```python
from build123d import *

# Parameters (mm, degrees)
BOSS_EXTRUDE1_DEPTH = 20
FILLET1_R           = 0.2
SKETCH2_R           = 2.7
CUT_EXTRUDE1_DEPTH  = 3.2
SKETCH3_R           = 2.7
CUT_EXTRUDE2_DEPTH  = 3.2


with BuildPart() as part:
    # Sketch1 → Boss-Extrude1 (new body)
    with BuildSketch(Plane.XY):
        with BuildLine():
            Line((5.679190751, 0), (19, 0))
            ThreePointArc((19, 0), (19.707106781, 0.292893219), (20, 1))
            Line((20, 1), (20, 2.2))
            ThreePointArc((20, 2.2), (19.707106781, 2.907106781), (19, 3.2))
            Line((19, 3.2), (5.2, 3.2))
            ThreePointArc((5.2, 3.2), (3.785786438, 3.785786438), (3.2, 5.2))
            Line((3.2, 5.2), (3.2, 19))
            ThreePointArc((3.2, 19), (2.907106781, 19.707106781), (2.2, 20))
            Line((2.2, 20), (1, 20))
            ThreePointArc((1, 20), (0.292893219, 19.707106781), (0, 19))
            Line((0, 19), (0, 2))
            ThreePointArc((0, 2), (0.585786438, 0.585786438), (2, 0))
            Line((2, 0), (5.679190751, 0))
        make_face()
    extrude(amount=BOSS_EXTRUDE1_DEPTH)

    # Fillet1
    fillet1_edges = [part.edges().sort_by_distance(p)[0] for p in [
        (2.907106781, 19.707106781, 20),
        (12.1, 3.2, 0),
        (19.707106781, 2.907106781, 0),
        (20, 1.6, 0),
        (19.707106781, 0.292893219, 0),
        (10.5, 0, 0),
        (0.585786438, 0.585786438, 0),
        (0, 10.5, 0),
        (0.292893219, 19.707106781, 0),
        (1.6, 20, 0),
        (1.6, 20, 20),
        (2.907106781, 19.707106781, 0),
        (3.2, 12.1, 0),
        (3.785786438, 3.785786438, 0),
        (0.292893219, 19.707106781, 20),
        (0, 10.5, 20),
        (0.585786438, 0.585786438, 20),
        (10.5, 0, 20),
        (19.707106781, 0.292893219, 20),
        (20, 1.6, 20),
        (19.707106781, 2.907106781, 20),
        (3.785786438, 3.785786438, 20),
        (12.1, 3.2, 20),
        (3.2, 12.1, 20),
    ]]
    fillet(fillet1_edges, radius=FILLET1_R)

    # Sketch2 → Cut-Extrude1 (cut)
    with BuildSketch(Plane.ZY):
        with Locations((10, 10)):
            Circle(SKETCH2_R)
    extrude(amount=-CUT_EXTRUDE1_DEPTH, mode=Mode.SUBTRACT)

    # Sketch3 → Cut-Extrude2 (cut)
    with BuildSketch(Plane.XZ):
        with Locations(Location((10, 10, 0), (0, 0, 270))):
            Circle(SKETCH3_R)
    extrude(amount=-CUT_EXTRUDE2_DEPTH, mode=Mode.SUBTRACT)


solid = part.part
```
Can you work these out from the model? Positions are in its coordinate system, mm. A direction names the side the tool comes from. Coordinates: 2 decimals unless noted, no trailing zeros. Loops run counter-clockwise (first coordinate to the right, second up) from the corner with the lowest first, then second, coordinate; pieces in that order, holes last. Notation, with made-up numbers: (20, 73.25) -> (26, 73.25) arc R13 cw to (26, 79.25) -> close; hole circle Ø9 at (-35, 74). An arc over 180 degrees is marked (long way). Put each result on its own line as item: value. Start each with the question number.
Q1. For faces 4 (the face through (14, 3.2, 10)), 5 (the face through (19.699, 0.285, 9.863)), which set-ups out of +Z, -Z, +X, -X, +Y, -Y let a thin tool reach every point of the face, with its end or its side?
Q2. I'm going to push flat-ended pins straight in: P1, Ø4.5, axis at y = 10, z = 10, coming from the -X side; P2, Ø2, axis at x = 11, z = 16.5, coming from the +Y side; P3, Ø5, axis at y = 17, z = 12.5, coming from the -X side; P4, Ø11, axis at y = 14.5, z = 12, coming from the +X side. Where does each tip first touch, or does it pass through?
Q3. I want a section at C-C (z = 10). Write out the boundary of the cut face in (x, y), plus the area to 3 significant figures.
Q4. I want a section at A-A (y = 10). Write out the boundary of the cut face in (x, z), plus the area to 3 significant figures.
Q5. I want a section at D-D (x = 7). Write out the boundary of the cut face in (y, z).
Q6. If I drill on line 1 (Y direction, x = 2.2, z = 10); line 2 (X direction, y = 11, z = 16), over which ranges is the centre line in solid material (lowest first)? Write a range as [from, to].
Q7. Thinking about a two-plate mould opening in X: for faces 1 (the face through (12.277, 1.578, 8.548)), 2 (the face through (2, 20, 10)), 3 (the face through (0.57, 0.6, 9.86)), which applies, pulls with the +X half, pulls with the -X half, needs draft (parallel to the pull), parting line crosses it, or undercut?
Taken from the geometry:
1. face 4: +Z, -Z, +X, +Y
1. face 5: +Z, -Z, +X, -Y
2. P1: passes through
2. P2: stops at y = 3.2
2. P3: stops at x = 0
2. P4: stops at x = 3.2
3. outline: (0, 2) arc R2 ccw to (2, 0) -> (7.3, 0) -> (7.3, 3.2) -> (5.2, 3.2) arc R2 cw to (3.2, 5.2) -> (3.2, 7.3) -> (0, 7.3) -> close; (0, 12.7) -> (3.2, 12.7) -> (3.2, 19) arc R1 ccw to (2.2, 20) -> (1, 20) arc R1 ccw to (0, 19) -> close; (12.7, 0) -> (19, 0) arc R1 ccw to (20, 1) -> (20, 2.2) arc R1 ccw to (19, 3.2) -> (12.7, 3.2) -> close
3. area: 82.3 mm2
4. outline: (0, 0.2) arc R0.2 ccw to (0.2, 0) -> (3, 0) arc R0.2 ccw to (3.2, 0.2) -> (3.2, 7.3) -> (0, 7.3) -> close; (0, 12.7) -> (3.2, 12.7) -> (3.2, 19.8) arc R0.2 ccw to (3, 20) -> (0.2, 20) arc R0.2 ccw to (0, 19.8) -> close
4. area: 46.7 mm2
5. outline: (0, 0.2) arc R0.2 ccw to (0.2, 0) -> (3, 0) arc R0.2 ccw to (3.2, 0.2) -> (3.2, 19.8) arc R0.2 ccw to (3, 20) -> (0.2, 20) arc R0.2 ccw to (0, 19.8) -> close
6. line 1: y = [0, 7.3], [12.7, 20]
6. line 2: x = [0, 3.2]
7. face 1: undercut
7. face 2: needs draft
7. face 3: pulls with the -X half
